Part model, mm, in its own coordinate system. A direction names the side the tool comes from. Give positions to 0.01 mm unless a question says otherwise; leave off trailing zeros. Loops run counter-clockwise (first coordinate to the right, second up) from the corner with the lowest first, then second, coordinate; pieces in that order, holes last. Notation, with made-up numbers: M -31,7.5 L -12,7.5 A20 cw -12,34.5 Z; hole C 47,-30 d8. An arc over 180 degrees is marked long. Answer in a Markdown table with one row per item.
from build123d import *

# Parameters (mm, degrees)
F0_R     = 7.874
F1_DEPTH = 10.922
F2_W     = 52.578
F2_H     = 10.922
F3_DEPTH = 33.528
F4_SIZE2 = 16.5711074263
F4_SIZE  = 28.702
F6_DEPTH = 10.923


with BuildPart() as f1:
    # F0 (on Front) → F1 (new body)
    with BuildSketch(Plane.XZ):
        Polygon((-46.3958915723, 58.6556293481), (-78.1458915723, 58.6556293481), (-78.1458915723, -11.0481244944), (49.1894248783, -11.0481244944), (49.1894248783, 33.0436209969), align=None)
        with Locations((30.1394248783, 8.0018755056)):
            Circle(F0_R, mode=Mode.SUBTRACT)
    extrude(amount=F1_DEPTH)

    # F2 (on face) → F3 (join)
    with BuildSketch(Plane.XZ.offset(10.922)):
        Polygon((-67.2238915723, 39.7518755056), (-78.1458915723, 39.7518755056), (-78.1458915723, -11.0481244944), (-67.2238915723, -11.0481244944), (-67.2238915723, -0.1261244944), align=None)
        with Locations((-40.9348915723, -5.5871244944)):
            Rectangle(F2_W, F2_H)
    extrude(amount=F3_DEPTH)

    # F4
    f4_edges = [f1.edges().sort_by_distance(p)[0] for p in [
        (-72.684892, -44.45, 39.751876),
    ]]
    f4_side = f1.faces().sort_by_distance((-68.037088, -44.45, 19.812876))[0]
    chamfer(f4_edges, length=F4_SIZE, length2=F4_SIZE2, reference=f4_side)

    # F5 (on face) → F6 (cut, through all)
    with BuildSketch(Plane.XY.offset(-0.1261244944)):
        Polygon((-14.6458915723, -10.922), (-67.2238915723, -44.45), (-14.6458915723, -44.45), align=None)
    extrude(amount=-F6_DEPTH, mode=Mode.SUBTRACT)


solid = f1.part
(1) Which spindle directions (+Z, -Z, +X, -X, +Y, -Y) get a long thin tool onto all of the face, cutting with end or side? Do faces 1 (the face through (-73, -19, 39.752)), 2 (the face through (-78.146, -17, 17)), 3 (the face through (-67.224, -24, 20)). Say none if no direction does.
Recorded:
| item | result |
|---|---|
| face 1 | +Z, +X, -X, -Y |
| face 2 | +Z, -Z, -X, +Y, -Y |
| face 3 | +Z, +X, -Y |
(2) Drill centre lines: line 1 along Y through (x, z) = (-23, 3); line 2 along Z through (x, y) = (-57.5, -24); line 3 along X through (y, z) = (-32, 27.5). Where is each one in solid material? Low to high.
Recorded:
| item | result |
|---|---|
| line 1 | y = -10.92 to 0 |
| line 2 | z = -11.05 to -0.13 |
| line 3 | x = -78.15 to -67.22 |
(3) Pull direction Z, two halves, no side cores. Call faces 4 (the face through (49.189, -5, 11)), 5 (the face through (2.07, -5.38, 45.67)), 6 (the face through (22.273, -5.385, 8.348)): +Z half, -Z half, draft (parallel to the pull), parting line (faces both ways), or undercut.
Recorded:
| item | result |
|---|---|
| face 4 | draft |
| face 5 | +Z half |
| face 6 | undercut |
(4) Saw through at A-A (z = 14.5). Write the cut outline in (x, y).
Recorded:
| item | result |
|---|---|
| outline | M -78.15,-42.46 L -67.22,-42.46 L -67.22,-10.92 L 25.69,-10.92 L 25.69,0 L -78.15,0 Z; M 34.59,-10.92 L 49.19,-10.92 L 49.19,0 L 34.59,0 Z |
(5) Pin check, flat tips, straight feed: pin 1 Ø17 at (y, z) = (-32, 19.5) entering from +X; pin 2 Ø5.5 at (x, y) = (-75.5, -15.5) entering from +Z; pin 3 Ø8 at (x, z) = (-60, 30) entering from -Y. Stop position of each tip, or through.
Recorded:
| item | result |
|---|---|
| pin 1 | stops at x = -67.22 |
| pin 2 | stops at z = 39.75 |
| pin 3 | stops at y = -10.92 |
(6) Saw through at C-C (z = -4.5). Write the cut outline in (x, y).
Recorded:
| item | result |
|---|---|
| outline | M -78.15,-44.45 L -67.22,-44.45 L -14.65,-10.92 L 49.19,-10.92 L 49.19,0 L -78.15,0 Z |
(7) Saw through at B-B (y = -9). Write the cut outline in (x, z), plus the area to 3 significant figures.
Recorded:
| item | result |
|---|---|
| outline | M -78.15,-11.05 L 49.19,-11.05 L 49.19,33.04 L -46.4,58.66 L -78.15,58.66 Z; hole C 30.14,8 d15.75 |
| area | 7,460 mm^2 |
(8) Saw through at D-D (x = -44). Write the cut outline in (y, z), plus the area to 3 significant figures.
Recorded:
| item | result |
|---|---|
| outline | M -29.64,-11.05 L 0,-11.05 L 0,58.01 L -10.92,58.01 L -10.92,-0.13 L -29.64,-0.13 Z |
| area | 959 mm^2 |
